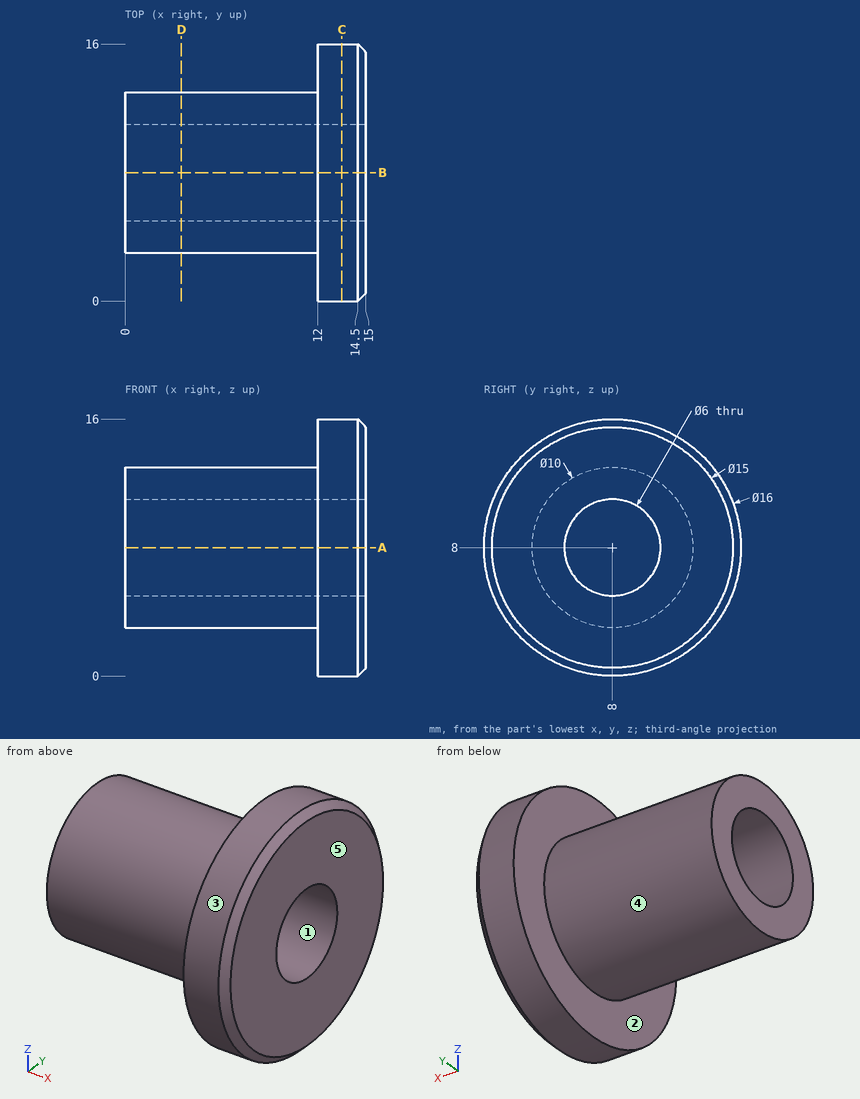
Answer from the drawing. Dimensions are ordinates in mm from the lowest x, y and z of the part. A direction names the side the tool comes from. Coordinates: 2 decimals unless noted, no trailing zeros. Loops run counter-clockwise (first coordinate to the right, second up) from the corner with the lowest first, then second, coordinate; pieces in that order, holes last.
1) Flat-ended cylindrical pins translate along their axes: pin 1 (8 mm diameter, centred on x = 12.5, y = 7, fed in from -Z); pin 2 (8 mm diameter, centred on x = 6.5, z = 8, fed in from -Y); pin 3 (1.5 mm diameter, centred on x = 4, z = 9.5, fed in from +Y); pin 4 (2 mm diameter, centred on x = 5.5, y = 12, fed in from -Z). Find the tip coordinate at first contact, or state that the pin passes through.
Results:
pin 1: stops at z = 0
pin 2: stops at y = 3
pin 3: stops at y = 12.94
pin 4: stops at z = 4
2) For a pull along Z with two mould halves and no side action, classify the marked faces 1, 2 and 3 as +Z half, -Z half, draft (parallel to the pull), parting line (faces both ways), or undercut.
Results:
face 1: undercut
face 2: draft
face 3: parting line
3) Section D-D (x = 3.5) is taken. Give the vertices of the cut face in (y, z).
Results:
outline: circle Ø10 at (8, 8); hole circle Ø6 at (8, 8)
4) Section C-C (x = 13.5) is taken. Give the vertices of the cut face in (y, z).
Results:
outline: circle Ø16 at (8, 8); hole circle Ø6 at (8, 8)
5) For the marked faces 4 and 5, determine the directions among +Z, -Z, +X, -X, +Y, -Y from which every point of the face is accessible in a straight line to the end or side of a thin tool.
Results:
face 4: -X
face 5: +Z, -Z, +X, +Y, -Y
6) Section A-A (z = 8) is taken. Give the vertices of the cut face in (x, y).
Results:
outline: (0, 3) - (12, 3) - (12, 0) - (14.5, 0) - (15, 0.5) - (15, 5) - (0, 5) - close; (0, 11) - (15, 11) - (15, 15.5) - (14.5, 16) - (12, 16) - (12, 13) - (0, 13) - close
7) Consider probe 1 along Y at (x, z) = (4, 8); probe 2 along X at (y, z) = (12.25, 2); probe 3 along Y at (x, z) = (8, 12). Determine where each line is inside the solid, lowest interval first.
Results:
probe 1: y = 3 to 5, 11 to 13
probe 2: x = 12 to 15
probe 3: y = 5 to 11
